from build123d import *

# Parameters (mm, degrees)
EXTRUDE_1_DEPTH     = 50
SKETCH_2_R          = 1.6
CUT_EXTRUDE_1_DEPTH = 4
SKETCH_3_W          = 50
SKETCH_3_H          = 3
CUT_EXTRUDE_2_DEPTH = 13.5
SKETCH_4_R          = 1.6
CUT_EXTRUDE_3_DEPTH = 26


with BuildPart() as part:
    # ｽｹｯﾁ1 → ﾎﾞｽ - 押し出し1 (new body)
    with BuildSketch(Plane(origin=(0, 0, 0), x_dir=(0, 0, -1), z_dir=(1, 0, 0))):
        Polygon((0, 50), (25, 50), (25, 47), (3, 47), (3, 0), (0, 0), align=None)
    extrude(amount=EXTRUDE_1_DEPTH)

    # ｽｹｯﾁ2 → ｶｯﾄ - 押し出し1 (cut, through all)
    with BuildSketch(Plane.XZ.offset(-47)):
        with Locations((8.5, -9)):
            Circle(SKETCH_2_R)
        with Locations((8.5, -21)):
            Circle(SKETCH_2_R)
        with Locations((41.5, -9)):
            Circle(SKETCH_2_R)
        with Locations((41.5, -21)):
            Circle(SKETCH_2_R)
    extrude(amount=-CUT_EXTRUDE_1_DEPTH, mode=Mode.SUBTRACT)

    # ｽｹｯﾁ3 → ｶｯﾄ - 押し出し2 (cut)
    with BuildSketch(Plane.XZ):
        with Locations((25, -1.5)):
            Rectangle(SKETCH_3_W, SKETCH_3_H)
    extrude(amount=-CUT_EXTRUDE_2_DEPTH, mode=Mode.SUBTRACT)

    # ｽｹｯﾁ4 → ｶｯﾄ - 押し出し3 (cut, through all)
    with BuildSketch(Plane.XY):
        with Locations((17.5, 22)):
            Circle(SKETCH_4_R)
        with Locations((32.5, 22)):
            Circle(SKETCH_4_R)
    extrude(amount=-CUT_EXTRUDE_3_DEPTH, mode=Mode.SUBTRACT)


solid = part.part
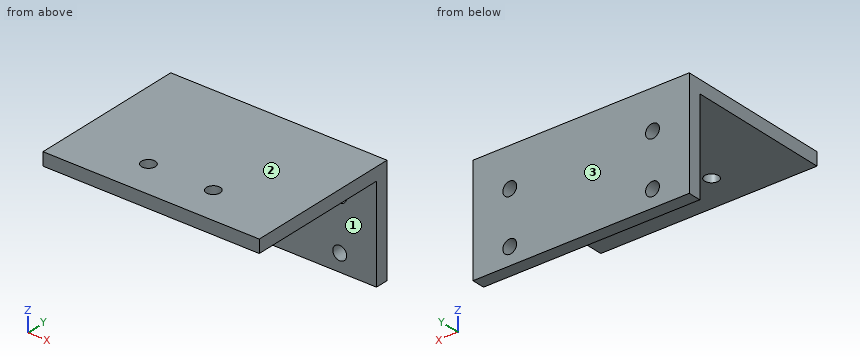
CAD build for the part. Positions are in the model's coordinates, mm. Face numbers are marked on the shaded views. Coordinates: 2 decimals unless noted, no trailing zeros. Write each loop counter-clockwise with the first axis right and the second up, starting at its lowest first coordinate (ties: lowest second). Pieces come first, ordered by that corner, then holes. Notation, with made-up numbers: M -26.75,85.5 L 24.25,85.5 A20 cw 24.25,99.5 Z; hole C 41,87 d6. An arc over 180 degrees is marked long. Answer as a JSON object with one key per item and string values. Group by question number.
1) Wall check: line 1 (Z direction, x = 8.5, y = 48.45); line 2 (Y direction, x = 32.5, z = -1.25); line 3 (Z direction, x = 8, y = 49). Give the ranges that are in metal, low to high. Write a range as from..to.
2) Pin check, flat tips, straight feed: pin 1 Ø2.5 at (x, y) = (17.5, 22) entering from -Z; pin 2 Ø12 at (x, z) = (30.5, -10.5) entering from -Y; pin 3 Ø12 at (x, y) = (27.5, 32.5) entering from -Z; pin 4 Ø2 at (x, y) = (19.5, 22.5) entering from +Z. Stop position of each tip, or through.
3) Saw through at B-B (x = 32.5). Write the cut outline in (y, z), plus the area to 3 significant figures.
4) Saw through at C-C (x = 8.5). Write the cut outline in (y, z), plus the area to 3 significant figures.
5) Mould opens along Y. For the marked faces 1, 2 and 3 say: +Y half, -Y half, draft (parallel to the pull), parting line (faces both ways), or undercut.
6) Saw through at A-A (y = 22). Write the cut outline in (x, z), plus the area to 3 significant figures.
7) Saw through at D-D (y = 48). Write the cut outline in (x, z).
Values follow:
{
 "1": {"line 1": "z = -25..-22.6, -19.4..-10.6, -7.4..0", "line 2": "y = 13.5..20.4, 23.6..50", "line 3": "z = -25..-22.52, -19.48..-10.52, -7.48..0"},
 "2": {"pin 1": "passes through", "pin 2": "stops at y = 47", "pin 3": "stops at z = -3", "pin 4": "stops at z = 0"},
 "3": {"outline": "M 13.5,-3 L 20.4,-3 L 20.4,0 L 13.5,0 Z; M 23.6,-3 L 47,-3 L 47,-25 L 50,-25 L 50,0 L 23.6,0 Z", "area": "166 mm2"},
 "4": {"outline": "M 13.5,-3 L 47,-3 L 47,-7.4 L 50,-7.4 L 50,0 L 13.5,0 Z; M 47,-25 L 50,-25 L 50,-22.6 L 47,-22.6 Z; M 47,-19.4 L 50,-19.4 L 50,-10.6 L 47,-10.6 Z", "area": "156 mm2"},
 "5": {"face 1": "-Y half", "face 2": "draft", "face 3": "+Y half"},
 "6": {"outline": "M 0,-3 L 15.9,-3 L 15.9,0 L 0,0 Z; M 19.1,-3 L 30.9,-3 L 30.9,0 L 19.1,0 Z; M 34.1,-3 L 50,-3 L 50,0 L 34.1,0 Z", "area": "131 mm2"},
 "7": {"outline": "M 0,-25 L 50,-25 L 50,0 L 0,0 Z; hole C 8.5,-21 d3.2; hole C 8.5,-9 d3.2; hole C 41.5,-21 d3.2; hole C 41.5,-9 d3.2"}
}
